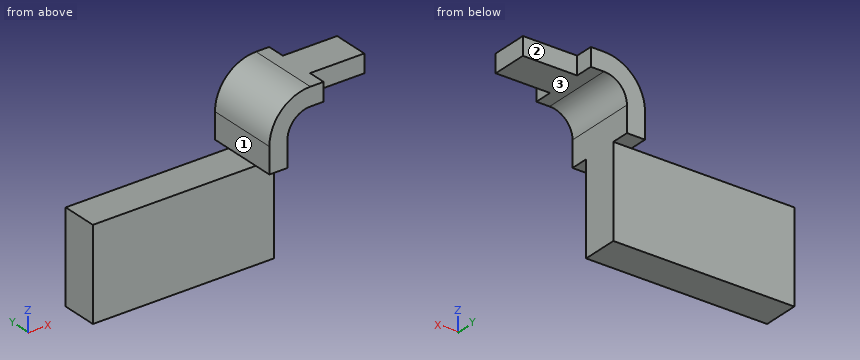
```python
from build123d import *

# Parameters (mm, degrees)
F1_DEPTH = 12.7
F2_DEPTH = 25.4
F0_W     = 38.1
F0_H     = 12.7
F3_DEPTH = 12.7


with BuildPart() as f1:
    # F0 (on Front) → F1 (new body, symmetric)
    with BuildSketch(Plane.XZ):
        Polygon((-63.5, 31.75), (-63.5, -31.75), (63.5, -31.75), (63.5, 31.75), (50.8, 31.75), align=None)
    extrude(amount=F1_DEPTH, both=True)

    # F0 (on Front) → F2 (join, symmetric)
    with BuildSketch(Plane.XZ):
        with BuildLine():
            Line((50.8, 31.75), (63.5, 31.75))
            Line((63.5, 31.75), (63.5, 49.721827))
            ThreePointArc((63.5, 49.721827), (68.214881, 61.104556), (79.59761, 65.819437))
            Line((79.59761, 65.819437), (88.861028, 65.819437))
            Line((88.861028, 65.819437), (88.861028, 78.519437))
            Line((88.861028, 78.519437), (79.59761, 78.519437))
            ThreePointArc((79.59761, 78.519437), (59.234625, 70.084812), (50.8, 49.721827))
            Line((50.8, 49.721827), (50.8, 31.75))
        make_face()
    extrude(amount=F2_DEPTH, both=True)

    # F0 (on Front) → F3 (join, symmetric)
    with BuildSketch(Plane.XZ):
        with Locations((107.911028, 72.169437)):
            Rectangle(F0_W, F0_H)
    extrude(amount=F3_DEPTH, both=True)


solid = f1.part
```
Check sheet for the modelled part. Datum: model origin and axes. Units: mm. Face numbers are marked on the shaded views. A direction names the side the tool comes from. Round coordinates to 2 decimals unless told otherwise and drop trailing zeros. Loops run counter-clockwise (first coordinate to the right, second up) from the corner with the lowest first, then second, coordinate; pieces in that order, holes last. Notation, with made-up numbers: (-0.75, 19) -> (32.25, 19) arc R27 ccw to (32.25, 55) -> close; hole circle Ø6 at (25, 10). An arc over 180 degrees is marked (long way). Write item = value, one per line. Start each with the question number.
1) Sectioned sample at B-B, the plane x = 84.5. Record the cut outline in (y, z), plus the area to 3 significant figures.
2) Gauge pin test, flat ends, axial feed: pin 1 Ø1 at (y, z) = (-4.5, 54.5) entering from -X; pin 2 Ø10 at (y, z) = (-8.5, 12.5) entering from +X; pin 3 Ø6.5 at (x, y) = (58, 17.5) entering from -Z. Record the tip position at first contact, or that the pin passes through.
3) Sectioned sample at A-A, the plane y = -16. Record the cut outline in (x, z), plus the area to 3 significant figures.
4) Sectioned sample at C-C, the plane z = 29. Record the cut outline in (x, y).
5) Thickness scan on probe 1 along Z at (x, y) = (113.5, -4.5); probe 2 along X at (y, z) = (3, -1); probe 3 along Z at (x, y) = (-4.5, -2.5). Record the ranges inside material, lowest first.
6) Set-up check for the marked faces 1, 2 and 3: record each of +Z, -Z, +X, -X, +Y, -Y from which the full face is reachable in a straight line by a thin tool's end or side.
Results are:
q1.outline = (-25.4, 65.82) -> (25.4, 65.82) -> (25.4, 78.52) -> (-25.4, 78.52) -> close
q1.area = 645 mm^2
q2.pin_1 = 51.12
q2.pin_2 = 63.5
q2.pin_3 = 31.75
q3.outline = (50.8, 31.75) -> (63.5, 31.75) -> (63.5, 49.72) arc R16.1 cw to (79.6, 65.82) -> (88.86, 65.82) -> (88.86, 78.52) -> (79.6, 78.52) arc R28.8 ccw to (50.8, 49.72) -> close
q3.area = 794 mm^2
q4.outline = (-63.5, -12.7) -> (63.5, -12.7) -> (63.5, 12.7) -> (-63.5, 12.7) -> close
q5.probe_1 = 65.82 to 78.52
q5.probe_2 = -63.5 to 63.5
q5.probe_3 = -31.75 to 31.75
q6.face_1 = +Z, -X, +Y, -Y
q6.face_2 = +Z, -Z, +X, +Y
q6.face_3 = -Z, +X, +Y, -Y
